Model file for the job. Use its own axes, mm. Face numbers are marked on the shaded views. A direction names the side the tool comes from. Coordinates: 2 decimals unless noted, no trailing zeros. Write each loop counter-clockwise with the first axis right and the second up, starting at its lowest first coordinate (ties: lowest second). Pieces come first, ordered by that corner, then holes. Notation, with made-up numbers: (-19.75, 24.25) - (-0.75, 24.25) arc R12 ccw to (-0.75, 41.25) - close; hole circle Ø11 at (59.5, 41). An arc over 180 degrees is marked (long way). Put each result on its own line as item: value. Start each with the question number.
1. Saw through at C-C, the plane z = 0. Write the cut outline in (x, y), plus the area to 4 significant figures.
2. Pull direction Z, two halves, no side cores. Call the marked faces 3, 4 and 5: released by +Z, released by -Z, zero draft, split by the parting line, or undercut.
3. Which spindle directions (+Z, -Z, +X, -X, +Y, -Y) get a long thin tool onto all of the face, cutting with end or side? Do the marked faces 1 and 2. Say none if no direction does.
4. Saw through at B-B, the plane x = 0. Write the cut outline in (y, z).
5. Drop flat-ended pins along their axis: P1, Ø12, axis at x = 10.5, y = 25, coming from the -Z side; P2, Ø10, axis at y = 13, z = -9, coming from the +X side; P3, Ø3, axis at x = -2, y = 15, coming from the -Z side. Give the stop position or say it passes through.
6. Saw through at D-D, the plane y = 11. Write the cut outline in (x, z).
7. Saw through at A-A, the plane y = 33. Write the cut outline in (x, z).
8. Drill centre lines: L1, parallel to X at y = 26, z = 0; L2, parallel to X at y = 15.5, z = -2; L3, parallel to X at y = 10, z = 0. Where is each one in solid material? Low to high. Write a range as from..to.
```python
from build123d import *

# Parameters (mm, degrees)
SKETCH1_R           = 16.25
BOSS_EXTRUDE1_DEPTH = 15
SKETCH2_R           = 11.65
BOSS_EXTRUDE2_DEPTH = 20
SKETCH3_R           = 16.25
SKETCH3_R_2         = 15.25
BOSS_EXTRUDE4_DEPTH = 20
SKETCH4_R           = 2.7
CUT_EXTRUDE1_DEPTH  = 30


with BuildPart() as part:
    # Sketch1 → Boss-Extrude1 (new body)
    with BuildSketch(Plane(origin=(0, 0, 0), x_dir=(1, 0, 0), z_dir=(0, 1, 0))):
        with Locations(Location((0, 0, 0), (0, 0, 270))):
            Circle(SKETCH1_R)
    extrude(amount=BOSS_EXTRUDE1_DEPTH)

    # Sketch2 → Boss-Extrude2 (add)
    with BuildSketch(Plane(origin=(0, 15, 0), x_dir=(1, 0, 0), z_dir=(0, 1, 0))):
        with Locations(Location((0, 0, 0), (0, 0, 270))):
            Circle(SKETCH2_R)
    extrude(amount=BOSS_EXTRUDE2_DEPTH)

    # Sketch3 → Boss-Extrude4 (add)
    with BuildSketch(Plane(origin=(0, 15, 0), x_dir=(1, 0, 0), z_dir=(0, 1, 0))):
        with Locations(Location((0, 0, 0), (0, 0, 270))):
            Circle(SKETCH3_R)
        with Locations(Location((0, 0, 0), (0, 0, 270))):
            Circle(SKETCH3_R_2, mode=Mode.SUBTRACT)
    extrude(amount=BOSS_EXTRUDE4_DEPTH)

    # Sketch4 → Cut-Extrude1 (cut)
    with BuildSketch(Plane(origin=(0, 35, 0), x_dir=(1, 0, 0), z_dir=(0, 1, 0))):
        with Locations(Location((0, 0, 0), (0, 0, 270))):
            Circle(SKETCH4_R)
    extrude(amount=-CUT_EXTRUDE1_DEPTH, mode=Mode.SUBTRACT)


solid = part.part
```
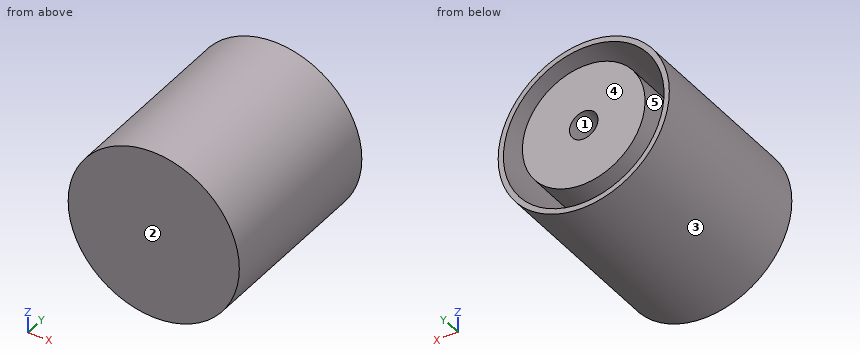
Final values:
1. outline: (-16.25, 0) - (16.25, 0) - (16.25, 35) - (15.25, 35) - (15.25, 15) - (11.65, 15) - (11.65, 35) - (2.7, 35) - (2.7, 5) - (-2.7, 5) - (-2.7, 35) - (-11.65, 35) - (-11.65, 15) - (-15.25, 15) - (-15.25, 35) - (-16.25, 35) - close
1. area: 831.5 mm²
2. face 3: split by the parting line
2. face 4: zero draft
2. face 5: undercut
3. face 1: +Y
3. face 2: +Z, -Z, +X, -X, -Y
4. outline: (0, -16.25) - (35, -16.25) - (35, -15.25) - (15, -15.25) - (15, -11.65) - (35, -11.65) - (35, -2.7) - (5, -2.7) - (5, 2.7) - (35, 2.7) - (35, 11.65) - (15, 11.65) - (15, 15.25) - (35, 15.25) - (35, 16.25) - (0, 16.25) - close
5. P1: stops at z = -15.61
5. P2: stops at x = 15.75
5. P3: stops at z = -16.24
6. outline: circle Ø32.5 at (0, 0); hole circle Ø5.4 at (0, 0)
7. outline: circle Ø32.5 at (0, 0); circle Ø23.3 at (0, 0); hole circle Ø30.5 at (0, 0); hole circle Ø5.4 at (0, 0)
8. L1: x = -16.25..-15.25, -11.65..-2.7, 2.7..11.65, 15.25..16.25
8. L2: x = -16.13..-15.12, -11.48..-1.81, 1.81..11.48, 15.12..16.13
8. L3: x = -16.25..-2.7, 2.7..16.25
